Autodesk Inventor part; units mm, degrees
ref_plane "YZ Plane" through (0, 0, 0) normal (1, 0, 0) x (0, 1, 0)
ref_plane "XZ Plane" through (0, 0, 0) normal (0, 1, 0) x (-1, 0, 0)
ref_plane "XY Plane" through (0, 0, 0) normal (0, 0, 1) x (1, 0, 0)
sketch "Sketch1" plane through (0, 0, 0) normal (0, 0, 1) x (1, 0, 0)
  line L0 (0, 0) -> (84, 0)
  line L1 (84, 0) -> (84, 15)
  line L2 (84, 15) -> (0, 15)
  line L3 (0, 15) -> (0, 0)
  dimension "d0" = 84
  dimension "d1" = 15
extrude "Plate1" add sketch "Sketch1" along normal blind 2
sketch "Sketch2" plane through (84, 2, 0) normal (0, -1, 0) x (1, 0, 0)
  line L0 (-84, 0) -> (0, 0)
  line L1 (0, 0) -> (0, 45)
  line L2 (0, 45) -> (-84, 45)
  line L3 (-84, 45) -> (-84, 0)
edge flange "Flange1" height 45 angle 90 thickness 2 bend radius 2 thickness toward (0, -1, 0) relief tear relief width 2 relief depth 1 edges at (42, 0, 2) wall of the first edge with corners at (0, 2, 0) (84, 2, 0) (84, 2, 45) (0, 2, 45)
bend "Bend1"
corner "Corner1"
sketch "Sketch3" plane through (0, 0, 0) normal (0, 0, -1) x (-1, 0, 0)
  line L0 (-84, 4) -> (0, 4)
  line L1 (0, 15) -> (0, 4)
  line L2 (-84, 15) -> (0, 15)
  line L3 (-84, 4) -> (-84, 15)
  circle A0 centre (-15, 9.5) radius 2.1
  circle A1 centre (-69, 9.5) radius 2.1
  point P0 (0, 0)
  point P1 (-84, 9.5)
  dimension "d13" = 15
  dimension "d14" = 15
  dimension "d15" = 4.2
extrude "Cut1" cut sketch "Sketch3" against normal blind 2 contours A0 | A1
fillet "Corner Round1" radius 2.5 4 edges at (84, 15, 1) (0, 15, 1) (84, 1, 45) (0, 1, 45)
sketch "Sketch5" plane through (0, 0, 4) normal (0, -1, 0) x (1, 0, 0)
  arc A0 (84, 38.5) -> (81.5, 41) centre (81.5, 38.5) ccw
  line L0 (2.5, 41) -> (81.5, 41)
  arc A1 (2.5, 41) -> (0, 38.5) centre (2.5, 38.5) ccw
  line L1 (0, 0) -> (0, 38.5)
  line L2 (0, 0) -> (84, 0)
  line L3 (84, 38.5) -> (84, 0)
  line L4 (84, -4) -> (84, 0)
  line L5 (0, 0) -> (0, -4)
  line L6 (84, -4) -> (0, -4)
  line L7 (81.5, -4) -> (2.5, -4)
  line L8 (45, 11) -> (39, 11)
  line L9 (39, 11) -> (39, -4)
  line L10 (39, -4) -> (45, -4)
  line L11 (45, -4) -> (45, 11)
  line L12 (45, 11) -> (39, -4) construction
  line L13 (39, 11) -> (45, -4) construction
  circle A2 centre (42, 11) radius 3
  point P0 (42, 3.5)
  point P1 (42, -4)
  dimension "d24" = 6
  dimension "d25" = 15
extrude "Cut3" cut sketch "Sketch5" against normal through all contours L11 L6 L9 L2 | L2 L9 A2 L11 | A2 L8 | L8 A2
equation "\"d14\" = d13"
equation "\"d16\" = Thickness"
equation "\"d26\" = Thickness"
equation "\"d2\" = Thickness"
equation "\"d3\" = BendReliefWidth"
equation "\"d4\" = BendReliefDepth"
equation "\"d5\" = MinimumRemnant"
equation "\"d6\" = TransitionRadius"
equation "\"d9\" = BendRadius"
equation "\"d10\" = CornerReliefSize"
equation "\"d11\" = GapSize"
equation "\"d12\" = JacobiRadiusSize"
equation "\"BendRadius\" = Thickness"
equation "\"BendReliefWidth\" = Thickness"
equation "\"BendReliefDepth\" = 0.5 * Thickness"
equation "\"CornerReliefSize\" = 4 * Thickness"
equation "\"MinimumRemnant\" = 2 * Thickness"
equation "\"TransitionRadius\" = BendRadius"
equation "\"JacobiRadiusSize\" = BendRadius"
equation "\"GapSize\" = Thickness"
properties part number "backing plate lidar" material "Aluminum 6061"
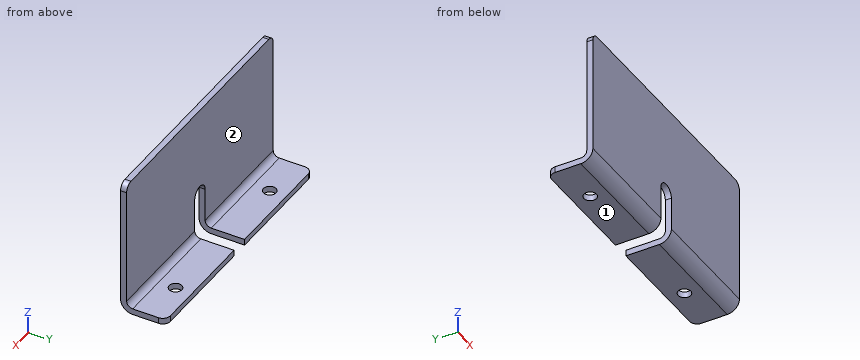
Geometry check sheet. Reference: the model listing, model coordinates, mm. Face numbers are marked on the shaded views. A direction names the side the tool comes from. Round coordinates to 2 decimals unless told otherwise and drop trailing zeros. Loops run counter-clockwise (first coordinate to the right, second up) from the corner with the lowest first, then second, coordinate; pieces in that order, holes last. Notation, with made-up numbers: (81, -23.75) - (100, -23.75) arc R30 cw to (100, 1.25) - close; hole circle Ø1 at (24.5, 8). An arc over 180 degrees is marked (long way). One line per question, with ' | ' between items. Start each with the question number.
1. Cross-section at C-C on x = 69. Record the cut outline in (y, z), then the cut area to 3 significant figures.
2. Cross-section at D-D on x = 52.5. Record the cut outline in (y, z), then the cut area to 3 significant figures.
3. Tool access check on the marked faces 1 and 2. Record the directions out of +Z, -Z, +X, -X, +Y, -Y that give a thin tool (end or side, any length) a straight path to the whole face; none if there is none.
4. Scan lines: line 1 (Z direction, x = 34.5, y = 11.5); line 2 (Y direction, x = 15, z = 1). Record each from-to range of solid material in increasing order. Write a range as [from, to].
5. Cross-section at A-A on y = 6.25. Record the cut outline in (x, z).
6. Depth check by flat-ended pin: pin 1 (6 mm diameter, centred on x = 75.5, y = 10.5, fed in from +Z); pin 2 (2 mm diameter, centred on x = 54.5, z = 4.5, fed in from +Y); pin 3 (5 mm diameter, centred on x = 40.5, y = 3.5, fed in from +Z); pin 4 (4 mm diameter, centred on x = 33, z = 32.5, fed in from +Y). Enter the tip coordinate at first touch or a pass-through.
Taken from the geometry:
1) outline: (0, 4) arc R4 ccw to (4, 0) - (7.4, 0) - (7.4, 2) - (4, 2) arc R2 cw to (2, 4) - (2, 45) - (0, 45) - close; (11.6, 0) - (15, 0) - (15, 2) - (11.6, 2) - close | area: 105 mm²
2) outline: (0, 4) arc R4 ccw to (4, 0) - (15, 0) - (15, 2) - (4, 2) arc R2 cw to (2, 4) - (2, 45) - (0, 45) - close | area: 113 mm²
3) face 1: -Z, +X, -X, +Y, -Y | face 2: +Z, +X, -X, +Y
4) line 1: [0, 2] | line 2: [1.35, 7.4], [11.6, 15]
5) outline: (0, 0) - (39, 0) - (39, 2) - (0, 2) - close; (45, 0) - (84, 0) - (84, 2) - (45, 2) - close
6) pin 1: z = 2 | pin 2: y = 2.06 | pin 3: z = 45 | pin 4: y = 2
